from build123d import *

# Parameters (mm, degrees)
CYLINDER104_R     = 1.1
CYLINDER104_DEPTH = 21
BOX102_W          = 2
BOX102_H          = 7
BOX102_DEPTH      = 21
BOX100_W          = 8.2
BOX100_H          = 7
BOX100_DEPTH      = 8.9


with BuildPart() as cylinder104:
    # Cylinder104 → Cylinder104 (new body)
    with BuildSketch(Plane(origin=(7, 18.5, 71), x_dir=(0, 0, -1), z_dir=(1, 0, 0))):
        Circle(CYLINDER104_R)
    extrude(amount=CYLINDER104_DEPTH)


with BuildPart() as cut068:
    # Box102 → Box102 (new body)
    with BuildSketch(Plane(origin=(12, 15, 53.1), x_dir=(1, 0, 0), z_dir=(0, 0, 1))):
        with Locations((1, 3.5)):
            Rectangle(BOX102_W, BOX102_H)
    extrude(amount=BOX102_DEPTH)

    # Cut068: cut Cylinder104
    add(cylinder104.part, mode=Mode.SUBTRACT)


with BuildPart() as cap:
    # Box100 → Box100 (new body)
    with BuildSketch(Plane(origin=(3.8, 15, 53.1), x_dir=(1, 0, 0), z_dir=(0, 0, 1))):
        with Locations((4.1, 3.5)):
            Rectangle(BOX100_W, BOX100_H)
    extrude(amount=BOX100_DEPTH)

    # Fusion088: union Cut068
    add(cut068.part)


solid = cap.part
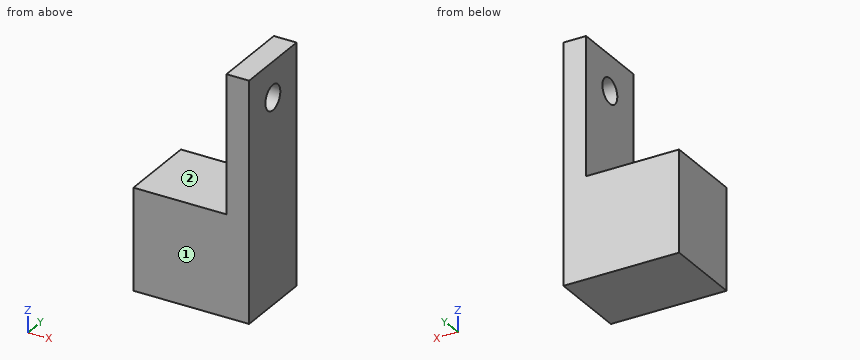
Work out the finished part from the listing and answer in its coordinate system (mm). Face numbers are marked on the shaded views. A direction names the side the tool comes from. Round coordinates to 2 decimals unless told otherwise and drop trailing zeros. Write each loop counter-clockwise with the first axis right and the second up, starting at its lowest first coordinate (ties: lowest second). Pieces come first, ordered by that corner, then holes.
1) A cutting plane is placed at A-A (z = 71). Give the vertices of the cut face in (x, y), plus the area to 3 significant figures.
2) A cutting plane is placed at C-C (y = 21.5). Give the vertices of the cut face in (x, z), plus the area to 3 significant figures.
3) Given pin 1 Ø2 at (y, z) = (18, 68) entering from -X; pin 2 Ø2 at (y, z) = (18.5, 71) entering from -X; pin 3 Ø2 at (x, y) = (7.5, 19) entering from +Z, each flat-ended and moving along its own axis, determine where each tip first touches the part or whether it passes through.
4) A cutting plane is placed at D-D (x = 9.75). Give the vertices of the cut face in (y, z), plus the area to 3 significant figures.
5) A tool of negligible diameter and unlimited length cuts with its end or side. For the marked faces 1 and 2, from which of +Z, -Z, +X, -X, +Y, -Y can it reach the whole face along a straight path? Write none if from no direction.
6) Straight lines are drawn through the part: line 1 (Y direction, x = 13.1, z = 71); line 2 (Z direction, x = 13.25, y = 18.5); line 3 (Z direction, x = 8.75, y = 16.75). For each, find the intervals that lie inside material, in ascending order.
7) A cutting plane is placed at B-B (y = 17.75). Give the vertices of the cut face in (x, z), plus the area to 3 significant figures.
Completed:
1. outline: (12, 15) - (14, 15) - (14, 17.4) - (12, 17.4) - close; (12, 19.6) - (14, 19.6) - (14, 22) - (12, 22) - close
1. area: 9.60 mm2
2. outline: (3.8, 53.1) - (14, 53.1) - (14, 74.1) - (12, 74.1) - (12, 62) - (3.8, 62) - close
2. area: 115 mm2
3. pin 1: stops at x = 12
3. pin 2: passes through
3. pin 3: stops at z = 62
4. outline: (15, 53.1) - (22, 53.1) - (22, 62) - (15, 62) - close
4. area: 62.3 mm2
5. face 1: +Z, -Z, +X, -X, -Y
5. face 2: +Z, -X, +Y, -Y
6. line 1: y = 15 to 17.4, 19.6 to 22
6. line 2: z = 53.1 to 69.9, 72.1 to 74.1
6. line 3: z = 53.1 to 62
7. outline: (3.8, 53.1) - (14, 53.1) - (14, 70.2) - (12, 70.2) - (12, 62) - (3.8, 62) - close; (12, 71.8) - (14, 71.8) - (14, 74.1) - (12, 74.1) - close
7. area: 112 mm2
